Read the model definition and answer for the solid it produces. Units are mm, in the model's axes. Face numbers are marked on the shaded views. Give positions to 0.01 mm unless a question says otherwise; leave off trailing zeros. Order: outer loops, then holes, each group sorted by start corner. A loop starts at its lowest first (then second) coordinate and runs counter-clockwise, first axis right, second up. Notation, with made-up numbers: (3, 74) -> (59, 74) arc R26 cw to (59, 102) -> close; hole circle Ø10 at (-24, 63). An arc over 180 degrees is marked (long way). Use one line per item in the form item = value.
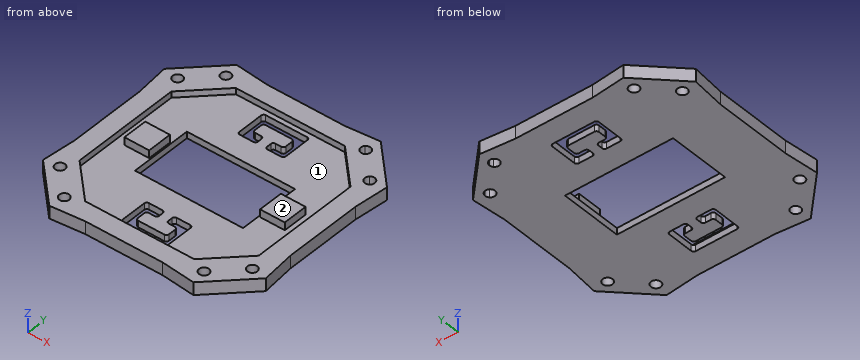
```python
from build123d import *

# Parameters (mm, degrees)
F0_R     = 1.6
F1_DEPTH = 4.1
F3_DEPTH = 2
F5_DEPTH = 2.101
F6_W     = 35
F6_H     = 20
F7_DEPTH = 2.101
F8_W     = 8
F8_H     = 8
F9_DEPTH = 2.5


with BuildPart() as f1:
    # F0 (on Top) → F1 (new body)
    with BuildSketch(Plane.XY):
        Polygon((0, 35), (0, 0), (26.870058, 26.870058), (29.698485, 29.698485), (23.334524, 36.062446), (12.5, 35), align=None)
        with BuildLine():
            ThreePointArc((24.227417, 31.112698), (24.105624, 30.500405), (23.758788, 29.981328))
            ThreePointArc((23.758788, 29.981328), (21.496046, 29.981328), (21.496046, 32.244069))
            ThreePointArc((21.496046, 32.244069), (23.23971, 32.590906), (24.227417, 31.112698))
        make_face(mode=Mode.SUBTRACT)
        Polygon((0, -35), (0, 0), (0, 35), (-12.5, 35), (-23.334524, 36.062446), (-36.062446, 23.334524), (-35, 12.5), (-35, -12.5), (-36.062446, -23.334524), (-23.334524, -36.062446), (-12.5, -35), align=None)
        with Locations((-22.627417, -31.112698)):
            Circle(F0_R, mode=Mode.SUBTRACT)
        with Locations((-31.112698, -22.627417)):
            Circle(F0_R, mode=Mode.SUBTRACT)
        with Locations((-31.112698, 22.627417)):
            Circle(F0_R, mode=Mode.SUBTRACT)
        with Locations((-22.627417, 31.112698)):
            Circle(F0_R, mode=Mode.SUBTRACT)
        Polygon((26.870058, 26.870058), (0, 0), (0, -35), (12.5, -35), (23.334524, -36.062446), (36.062446, -23.334524), (35, -12.5), (35, 12.5), (36.062446, 23.334524), (29.698485, 29.698485), align=None)
        with Locations((22.627417, -31.112698)):
            Circle(F0_R, mode=Mode.SUBTRACT)
        with Locations((31.112698, -22.627417)):
            Circle(F0_R, mode=Mode.SUBTRACT)
        with BuildLine():
            ThreePointArc((32.244069, 21.496046), (29.981328, 21.496046), (29.981328, 23.758788))
            ThreePointArc((29.981328, 23.758788), (31.724992, 24.105624), (32.712698, 22.627417))
            ThreePointArc((32.712698, 22.627417), (32.590906, 22.015124), (32.244069, 21.496046))
        make_face(mode=Mode.SUBTRACT)
    extrude(amount=F1_DEPTH)

    # F2 (on face) → F3 (cut)
    with BuildSketch(Plane.XY.offset(4.1)):
        Polygon((-29, 17.669048), (-29, 0), (0, 0), (0, 29), (-17.669048, 29), align=None)
        Polygon((0, 0), (-29, 0), (-29, -17.669048), (-17.669048, -29), (17.669048, -29), (29, -17.669048), (29, 17.669045), (17.669045, 29), (0, 29), align=None)
    extrude(amount=-F3_DEPTH, mode=Mode.SUBTRACT)

    # F4 (on face) → F5 (cut, through all)
    with BuildSketch(Plane.XY.offset(2.1)):
        with BuildLine():
            Line((6.7, 27.5), (0, 27.5))
            Line((0, 27.5), (0, 24.5))
            Line((0, 24.5), (4.2, 24.5))
            ThreePointArc((4.2, 24.5), (4.765685, 24.265685), (5, 23.7))
            Line((5, 23.7), (5, 21.3))
            ThreePointArc((5, 21.3), (4.765685, 20.734315), (4.2, 20.5))
            Line((4.2, 20.5), (2.3, 20.5))
            ThreePointArc((2.3, 20.5), (1.734315, 20.265685), (1.5, 19.7))
            Line((1.5, 19.7), (1.5, 18.3))
            ThreePointArc((1.5, 18.3), (1.734315, 17.734315), (2.3, 17.5))
            Line((2.3, 17.5), (6.7, 17.5))
            ThreePointArc((6.7, 17.5), (7.265685, 17.734315), (7.5, 18.3))
            Line((7.5, 18.3), (7.5, 26.7))
            ThreePointArc((7.5, 26.7), (7.265685, 27.265685), (6.7, 27.5))
        make_face()
        with BuildLine():
            Line((0, 24.5), (0, 27.5))
            Line((0, 27.5), (-6.7, 27.5))
            ThreePointArc((-6.7, 27.5), (-7.265685, 27.265685), (-7.5, 26.7))
            Line((-7.5, 26.7), (-7.5, 18.3))
            ThreePointArc((-7.5, 18.3), (-7.265685, 17.734315), (-6.7, 17.5))
            Line((-6.7, 17.5), (-2.3, 17.5))
            ThreePointArc((-2.3, 17.5), (-1.734315, 17.734315), (-1.5, 18.3))
            Line((-1.5, 18.3), (-1.5, 19.7))
            ThreePointArc((-1.5, 19.7), (-1.734315, 20.265685), (-2.3, 20.5))
            Line((-2.3, 20.5), (-4.2, 20.5))
            ThreePointArc((-4.2, 20.5), (-4.765685, 20.734315), (-5, 21.3))
            Line((-5, 21.3), (-5, 23.7))
            ThreePointArc((-5, 23.7), (-4.765685, 24.265685), (-4.2, 24.5))
            Line((-4.2, 24.5), (0, 24.5))
        make_face()
        with BuildLine():
            Line((-4.2, -20.5), (-2.3, -20.5))
            ThreePointArc((-2.3, -20.5), (-1.734315, -20.265685), (-1.5, -19.7))
            Line((-1.5, -19.7), (-1.5, -18.3))
            ThreePointArc((-1.5, -18.3), (-1.734315, -17.734315), (-2.3, -17.5))
            Line((-2.3, -17.5), (-6.7, -17.5))
            ThreePointArc((-6.7, -17.5), (-7.265685, -17.734315), (-7.5, -18.3))
            Line((-7.5, -18.3), (-7.5, -26.7))
            ThreePointArc((-7.5, -26.7), (-7.265685, -27.265685), (-6.7, -27.5))
            Line((-6.7, -27.5), (6.7, -27.5))
            ThreePointArc((6.7, -27.5), (7.265685, -27.265685), (7.5, -26.7))
            Line((7.5, -26.7), (7.5, -18.3))
            ThreePointArc((7.5, -18.3), (7.265685, -17.734315), (6.7, -17.5))
            Line((6.7, -17.5), (2.3, -17.5))
            ThreePointArc((2.3, -17.5), (1.734315, -17.734315), (1.5, -18.3))
            Line((1.5, -18.3), (1.5, -19.7))
            ThreePointArc((1.5, -19.7), (1.734315, -20.265685), (2.3, -20.5))
            Line((2.3, -20.5), (4.2, -20.5))
            ThreePointArc((4.2, -20.5), (4.765685, -20.734315), (5, -21.3))
            Line((5, -21.3), (5, -23.7))
            ThreePointArc((5, -23.7), (4.765685, -24.265685), (4.2, -24.5))
            Line((4.2, -24.5), (-4.2, -24.5))
            ThreePointArc((-4.2, -24.5), (-4.765685, -24.265685), (-5, -23.7))
            Line((-5, -23.7), (-5, -21.3))
            ThreePointArc((-5, -21.3), (-4.765685, -20.734315), (-4.2, -20.5))
        make_face()
    extrude(amount=-F5_DEPTH, mode=Mode.SUBTRACT)

    # F6 (on face) → F7 (cut, through all)
    with BuildSketch(Plane.XY.offset(2.1)):
        Rectangle(F6_W, F6_H)
    extrude(amount=-F7_DEPTH, mode=Mode.SUBTRACT)

    # F8 (on face) → F9 (join)
    with BuildSketch(Plane.XY.offset(2.1)):
        with Locations((-21.959, 0)):
            Rectangle(F8_W, F8_H)
        with Locations((21.959, 0)):
            Rectangle(F8_W, F8_H)
    extrude(amount=F9_DEPTH)


solid = f1.part
```
Item 1: Determine the mould class of the marked faces 1 and 2 for opening direction Y: +Y half, -Y half, draft (parallel to the pull), parting line (faces both ways), or undercut.
Checks:
face_1 = undercut
face_2 = draft
Item 2: The part is cut by section A-A on x = 0. Give the vertices of the cut face in (y, z), and give its area (3 significant figures).
Checks:
outline = (-35, 0) -> (-27.5, 0) -> (-27.5, 2.1) -> (-29, 2.1) -> (-29, 4.1) -> (-35, 4.1) -> close; (-24.5, 0) -> (-10, 0) -> (-10, 2.1) -> (-24.5, 2.1) -> close; (10, 0) -> (24.5, 0) -> (24.5, 2.1) -> (10, 2.1) -> close; (27.5, 0) -> (35, 0) -> (35, 4.1) -> (29, 4.1) -> (29, 2.1) -> (27.5, 2.1) -> close
area = 116 mm²
Item 3: The part is cut by section D-D on y = 2.5. Give the vertices of the cut face in (x, z).
Checks:
outline = (-35, 0) -> (-17.5, 0) -> (-17.5, 2.1) -> (-17.96, 2.1) -> (-17.96, 4.6) -> (-25.96, 4.6) -> (-25.96, 2.1) -> (-29, 2.1) -> (-29, 4.1) -> (-35, 4.1) -> close; (17.5, 0) -> (35, 0) -> (35, 4.1) -> (29, 4.1) -> (29, 2.1) -> (25.96, 2.1) -> (25.96, 4.6) -> (17.96, 4.6) -> (17.96, 2.1) -> (17.5, 2.1) -> close
Item 4: Given pin 1 Ø2.5 at (x, y) = (31.11, -22.63) entering from +Z; pin 2 Ø1.7 at (y, z) = (22, 1.5) entering from +X; pin 3 Ø2 at (x, z) = (21.5, 3) entering from -Y; pin 4 Ø2 at (y, z) = (-2, 2) entering from +X, each flat-ended and moving along its own axis, determine where each tip first touches the part or whether it passes through.
Checks:
pin_1 = through
pin_2 = 36.01
pin_3 = -35.98
pin_4 = 35
Item 5: The part is cut by section C-C on y = -7.5. Give the vertices of the cut face in (x, z), and give its area (3 significant figures).
Checks:
outline = (-35, 0) -> (-17.5, 0) -> (-17.5, 2.1) -> (-29, 2.1) -> (-29, 4.1) -> (-35, 4.1) -> close; (17.5, 0) -> (35, 0) -> (35, 4.1) -> (29, 4.1) -> (29, 2.1) -> (17.5, 2.1) -> close
area = 97.5 mm²
Item 6: The part is cut by section B-B on x = 9.5. Give the vertices of the cut face in (y, z), and give its area (3 significant figures).
Checks:
outline = (-35, 0) -> (-10, 0) -> (-10, 2.1) -> (-29, 2.1) -> (-29, 4.1) -> (-35, 4.1) -> close; (10, 0) -> (35, 0) -> (35, 4.1) -> (29, 4.1) -> (29, 2.1) -> (10, 2.1) -> close
area = 129 mm²
Item 7: Straight lines are drawn through the part: L1, parallel to X at y = -1, z = 2.9; L2, parallel to Y at x = 3, z = 2.05; L3, parallel to X at y = 10.5, z = 2.8. For each, find the intervals that lie inside material, in ascending order. Write a range as from..to.
Checks:
L1 = -35..-29, -25.96..-17.96, 17.96..25.96, 29..35
L2 = -35..-27.5, -24.5..-20.5, -17.5..-10, 10..17.5, 20.5..24.5, 27.5..35
L3 = -35..-29, 29..35
